from build123d import *

# Parameters (mm, degrees)
F0_W        = 60
F0_H        = 2.8
F0_W_2      = 2.8
F0_H_2      = 60
F0_W_3      = 7.9
F0_H_3      = 7.9
F1_DEPTH    = 75.8
F2_DEPTH    = 70.2
F3_DEPTH    = 75.8
F4_DEPTH    = 2.8
F5_T1_DEPTH = 2.8
F5_T3_DEPTH = 106.4
F5_T5_DEPTH = 103.6


# Not quite as in the source:
# - a fillet or chamfer that OpenCascade refuses, or shapes differently, is made with other operations: its cross-section is extruded or revolved along the edge and cut away or added


with BuildPart() as f1:
    # F0 (on Top) → F1 (new body)
    with BuildSketch(Plane.XY):
        with Locations((0, 39.3)):
            Rectangle(F0_W, F0_H)
        Polygon((-40.7, 30), (-37.9, 30), (-37.9, 37.9), (-30, 37.9), (-30, 40.7), (-40.7, 40.7), align=None)
        Polygon((37.9, 37.9), (37.9, 30), (40.7, 30), (40.7, 40.7), (30, 40.7), (30, 37.9), align=None)
        with Locations((39.3, 0)):
            Rectangle(F0_W_2, F0_H_2)
        Polygon((37.9, -30), (37.9, -37.9), (30, -37.9), (30, -40.7), (40.7, -40.7), (40.7, -30), align=None)
        with Locations((0, -39.3)):
            Rectangle(F0_W, F0_H)
        Polygon((-30, -40.7), (-30, -37.9), (-37.9, -37.9), (-37.9, -30), (-40.7, -30), (-40.7, -40.7), align=None)
        with Locations((-39.3, 0)):
            Rectangle(F0_W_2, F0_H_2)
        with Locations((33.95, -33.95)):
            Rectangle(F0_W_3, F0_H_3)
        with Locations((33.95, 33.95)):
            Rectangle(F0_W_3, F0_H_3)
        with Locations((-33.95, 33.95)):
            Rectangle(F0_W_3, F0_H_3)
        with Locations((-33.95, 0)):
            Rectangle(F0_W_3, F0_H_2)
        with Locations((33.95, 0)):
            Rectangle(F0_W_3, F0_H_2)
        with Locations((-33.95, -33.95)):
            Rectangle(F0_W_3, F0_H_3)
        with Locations((0, -33.95)):
            Rectangle(F0_W, F0_H_3)
        with Locations((0, 33.95)):
            Rectangle(F0_W, F0_H_3)
    extrude(amount=F1_DEPTH)

    # F0 (on Top) → F2 (cut)
    with BuildSketch(Plane.XY):
        Polygon((-40.7, 30), (-37.9, 30), (-37.9, 37.9), (-30, 37.9), (-30, 40.7), (-40.7, 40.7), align=None)
        with Locations((-33.95, 33.95)):
            Rectangle(F0_W_3, F0_H_3)
        with Locations((-39.3, 0)):
            Rectangle(F0_W_2, F0_H_2)
        with Locations((-33.95, 0)):
            Rectangle(F0_W_3, F0_H_2)
        Polygon((-30, -40.7), (-30, -37.9), (-37.9, -37.9), (-37.9, -30), (-40.7, -30), (-40.7, -40.7), align=None)
        with Locations((-33.95, -33.95)):
            Rectangle(F0_W_3, F0_H_3)
        with Locations((0, -39.3)):
            Rectangle(F0_W, F0_H)
        with Locations((33.95, -33.95)):
            Rectangle(F0_W_3, F0_H_3)
        with Locations((33.95, 0)):
            Rectangle(F0_W_3, F0_H_2)
        with Locations((33.95, 33.95)):
            Rectangle(F0_W_3, F0_H_3)
        with Locations((0, 33.95)):
            Rectangle(F0_W, F0_H_3)
        with Locations((0, 39.3)):
            Rectangle(F0_W, F0_H)
        Polygon((37.9, 37.9), (37.9, 30), (40.7, 30), (40.7, 40.7), (30, 40.7), (30, 37.9), align=None)
        with Locations((39.3, 0)):
            Rectangle(F0_W_2, F0_H_2)
        Polygon((37.9, -30), (37.9, -37.9), (30, -37.9), (30, -40.7), (40.7, -40.7), (40.7, -30), align=None)
        with Locations((0, -33.95)):
            Rectangle(F0_W, F0_H_3)
    extrude(amount=F2_DEPTH, mode=Mode.SUBTRACT)

    # F0 (on Top) → F3 (join)
    with BuildSketch(Plane.XY):
        Polygon((-30, -40.7), (-30, -37.9), (-37.9, -37.9), (-37.9, -30), (-40.7, -30), (-40.7, -40.7), align=None)
        Polygon((37.9, -30), (37.9, -37.9), (30, -37.9), (30, -40.7), (40.7, -40.7), (40.7, -30), align=None)
        Polygon((37.9, 37.9), (37.9, 30), (40.7, 30), (40.7, 40.7), (30, 40.7), (30, 37.9), align=None)
        Polygon((-40.7, 30), (-37.9, 30), (-37.9, 37.9), (-30, 37.9), (-30, 40.7), (-40.7, 40.7), align=None)
    extrude(amount=F3_DEPTH)

    # F0 (on Top) → F4 (join)
    with BuildSketch(Plane.XY):
        Polygon((-30, -40.7), (-30, -37.9), (-37.9, -37.9), (-37.9, -30), (-40.7, -30), (-40.7, -40.7), align=None)
        with Locations((-33.95, -33.95)):
            Rectangle(F0_W_3, F0_H_3)
        with Locations((0, -33.95)):
            Rectangle(F0_W, F0_H_3)
        with Locations((0, -39.3)):
            Rectangle(F0_W, F0_H)
        Polygon((37.9, -30), (37.9, -37.9), (30, -37.9), (30, -40.7), (40.7, -40.7), (40.7, -30), align=None)
        with Locations((33.95, -33.95)):
            Rectangle(F0_W_3, F0_H_3)
        with Locations((39.3, 0)):
            Rectangle(F0_W_2, F0_H_2)
        with Locations((33.95, 0)):
            Rectangle(F0_W_3, F0_H_2)
        with Locations((33.95, 33.95)):
            Rectangle(F0_W_3, F0_H_3)
        Polygon((37.9, 37.9), (37.9, 30), (40.7, 30), (40.7, 40.7), (30, 40.7), (30, 37.9), align=None)
        with Locations((0, 33.95)):
            Rectangle(F0_W, F0_H_3)
        with Locations((0, 39.3)):
            Rectangle(F0_W, F0_H)
        with Locations((-33.95, 33.95)):
            Rectangle(F0_W_3, F0_H_3)
        Polygon((-40.7, 30), (-37.9, 30), (-37.9, 37.9), (-30, 37.9), (-30, 40.7), (-40.7, 40.7), align=None)
        with Locations((-39.3, 0)):
            Rectangle(F0_W_2, F0_H_2)
        with Locations((-33.95, 0)):
            Rectangle(F0_W_3, F0_H_2)
    extrude(amount=-F4_DEPTH)

    # F5: fillet of radius 5 on 3 edges, made by hand

    # F5_s2 → F5_t1 (join)
    with BuildSketch(Plane.YZ.offset(37.9)):
        with BuildLine():
            ThreePointArc((-25, 0), (-28.5355339059, 1.4644660941), (-30, 5))
            Line((-30, 5), (-30, 0))
            Line((-30, 0), (-25, 0))
        make_face()
    extrude(amount=F5_T1_DEPTH)

    # F5_s4 → F5_t3 (cut)
    with BuildSketch(Plane.YZ.offset(-53.2)):
        with BuildLine():
            ThreePointArc((40.7, 2.2), (39.2355339059, -1.3355339059), (35.7, -2.8))
            Line((35.7, -2.8), (40.7, -2.8))
            Line((40.7, -2.8), (40.7, 2.2))
        make_face()
    extrude(amount=F5_T3_DEPTH, mode=Mode.SUBTRACT)

    # F5_s6 → F5_t5 (cut)
    with BuildSketch(Plane.XY.offset(-15.3)):
        with BuildLine():
            ThreePointArc((40.7, 35.7), (39.2355339059, 39.2355339059), (35.7, 40.7))
            Line((35.7, 40.7), (40.7, 40.7))
            Line((40.7, 40.7), (40.7, 35.7))
        make_face()
    extrude(amount=F5_T5_DEPTH, mode=Mode.SUBTRACT)


solid = f1.part
Build history of the part. All positions in model axes, mm. A direction names the side the tool comes from. Round coordinates to 2 decimals unless told otherwise and drop trailing zeros. Write each loop counter-clockwise with the first axis right and the second up, starting at its lowest first coordinate (ties: lowest second). Pieces come first, ordered by that corner, then holes. Notation, with made-up numbers: (45, 42) - (74, 42) arc R28 ccw to (74, 78) - close; hole circle Ø5 at (68.25, 72). An arc over 180 degrees is marked (long way). One line per question, with ' | ' between items.
1. Mould opens along X. For faces 1 (the face through (-37.9, 34, 35)), 2 (the face through (-30, 0, -1)), 3 (the face through (39.27, 39.2, 35.95)), 4 (the face through (-39, 30, 35)) say: released by +X, released by -X, zero draft, split by the parting line, or undercut.
Results are:
face 1: undercut | face 2: undercut | face 3: released by +X | face 4: zero draft
2. Drop flat-ended pins along their axis: pin 1 Ø24.5 at (x, y) = (-10, 8.5) entering from +Z; pin 2 Ø2 at (y, z) = (39.5, 32.5) entering from +X; pin 3 Ø3 at (x, z) = (8, -2) entering from +Y. Give the stop position or say it passes through.
Results are:
pin 1: through | pin 2: x = 39.84 | pin 3: y = 39.91
3. Band-saw the part on C-C, the plane x = -13. Write the cut outline in (y, z).
Results are:
outline: (-40.7, -2.8) - (-30, -2.8) - (-30, 0) - (-40.7, 0) - close; (-40.7, 70.2) - (-30, 70.2) - (-30, 75.8) - (-40.7, 75.8) - close; (30, -2.8) - (35.7, -2.8) arc R5 ccw to (40.19, 0) - (30, 0) - close; (30, 70.2) - (40.7, 70.2) - (40.7, 75.8) - (30, 75.8) - close
4. Drill centre lines: line 1 along X through (y, z) = (31, 24); line 2 along X through (y, z) = (-13.5, 71.5). Where is each one in solid material? Low to high. Write a range as from..to.
Results are:
line 1: -40.7..-37.9, 37.9..40.7 | line 2: -40.7..-30, 30..40.7
5. Tool access for faces 5 (the face through (0, -30, 73)), 6 (the face through (39, 30, 35)), 7 (the face through (-34, 37.9, 35)): list every direction of +Z, -Z, +X, -X, +Y, -Y with a clear straight run to the whole face (end or side of a thin tool).
Results are:
face 5: +Z, -Z | face 6: +X, -X | face 7: none
6. Band-saw the part on D-D, the plane y = -18. Write the cut outline in (x, z), and give its area (3 significant figures).
Results are:
outline: (-40.7, -2.8) - (-30, -2.8) - (-30, 0) - (-40.7, 0) - close; (-40.7, 70.2) - (-30, 70.2) - (-30, 75.8) - (-40.7, 75.8) - close; (30, -2.8) - (40.7, -2.8) - (40.7, 0) - (30, 0) - close; (30, 70.2) - (40.7, 70.2) - (40.7, 75.8) - (30, 75.8) - close | area: 180 mm^2
7. Band-saw the part on B-B, the plane z = 49. Write the cut outline in (x, y), and give its area (3 significant figures).
Results are:
outline: (-40.7, -40.7) - (-30, -40.7) - (-30, -37.9) - (-37.9, -37.9) - (-37.9, -30) - (-40.7, -30) - close; (-40.7, 30) - (-37.9, 30) - (-37.9, 37.9) - (-30, 37.9) - (-30, 40.7) - (-40.7, 40.7) - close; (30, -40.7) - (40.7, -40.7) - (40.7, -30) - (37.9, -30) - (37.9, -37.9) - (30, -37.9) - close; (30, 37.9) - (37.9, 37.9) - (37.9, 30) - (40.7, 30) - (40.7, 35.7) arc R5 ccw to (35.7, 40.7) - (30, 40.7) - close | area: 203 mm^2
8. Band-saw the part on A-A, the plane y = 34. Write the cut outline in (x, z), and give its area (3 significant figures).
Results are:
outline: (-40.7, -2.8) - (40.7, -2.8) - (40.7, 75.8) - (-40.7, 75.8) - close; hole (-37.9, 0) - (37.9, 0) - (37.9, 70.2) - (-37.9, 70.2) - close | area: 1,080 mm^2
